Geometry check sheet. Reference: drawing and pictorial views, mm from the part's lowest x, y, z. A direction names the side the tool comes from. Give positions to 0.01 mm unless a question says otherwise; leave off trailing zeros. Write each loop counter-clockwise with the first axis right and the second up, starting at its lowest first coordinate (ties: lowest second). Pieces come first, ordered by that corner, then holes.
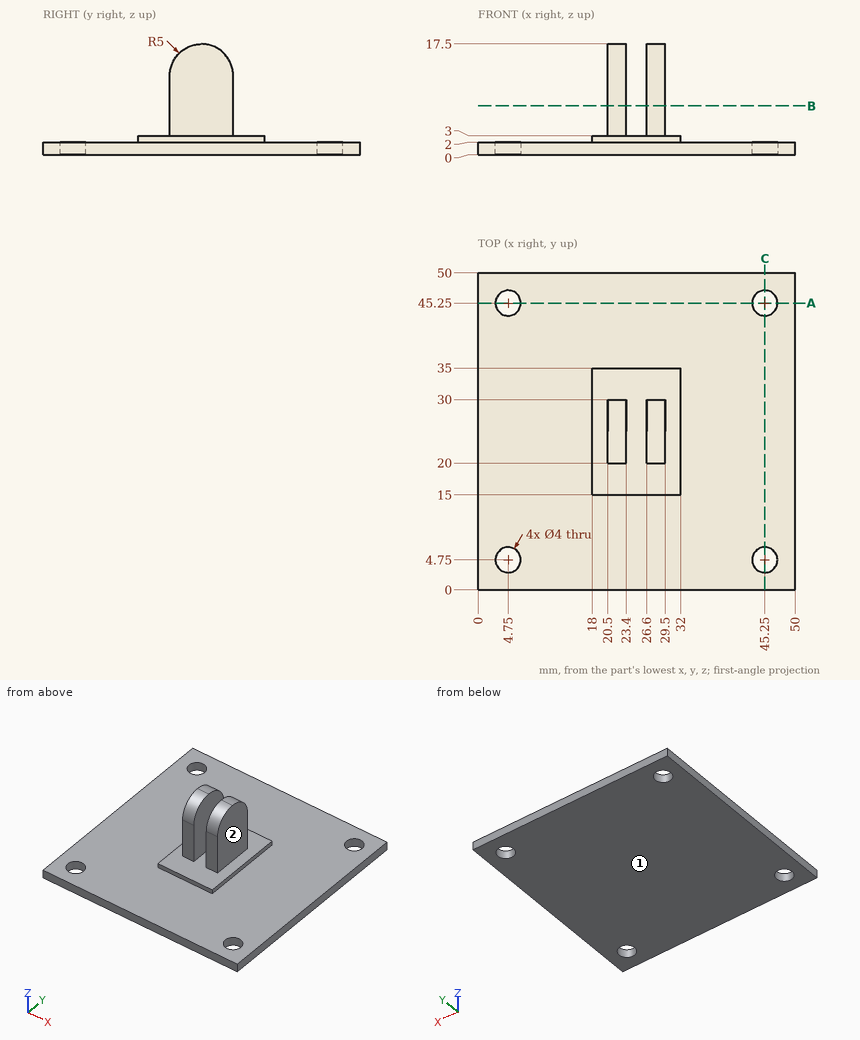
Item 1: Scan lines: line 1 along Y through (x, z) = (4.75, 1.4); line 2 along Z through (x, y) = (37, 6.5); line 3 along Z through (x, y) = (27.5, 34). Record each from-to range of solid material in increasing order.
Answer key:
line 1: y = 0 to 2.75, 6.75 to 43.25, 47.25 to 50
line 2: z = 0 to 2
line 3: z = 0 to 3
Item 2: Sectioned sample at A-A on y = 45.25. Record the cut outline in (x, z).
Answer key:
outline: (0, 0) - (2.75, 0) - (2.75, 2) - (0, 2) - close; (6.75, 0) - (43.25, 0) - (43.25, 2) - (6.75, 2) - close; (47.25, 0) - (50, 0) - (50, 2) - (47.25, 2) - close
Item 3: Sectioned sample at B-B on z = 7.75. Record the cut outline in (x, y), then the cut area to 3 significant figures.
Answer key:
outline: (20.5, 20) - (23.4, 20) - (23.4, 30) - (20.5, 30) - close; (26.6, 20) - (29.5, 20) - (29.5, 30) - (26.6, 30) - close
area: 58.0 mm2
Item 4: Depth check by flat-ended pin: pin 1 (8 mm diameter, centred on y = 27, z = 12.5, fed in from +X); pin 2 (2.5 mm diameter, centred on x = 22.5, z = 10, fed in from +Y); pin 3 (1.5 mm diameter, centred on x = 22, z = 7, fed in from -Y). Enter the tip coordinate at first touch or a pass-through.
Answer key:
pin 1: stops at x = 29.5
pin 2: stops at y = 30
pin 3: stops at y = 20
Item 5: Set-up check for the marked faces 1 and 2: record each of +Z, -Z, +X, -X, +Y, -Y from which the full face is reachable in a straight line by a thin tool's end or side.
Answer key:
face 1: -Z, +X, -X, +Y, -Y
face 2: +Z, +X, +Y, -Y
